Geometry: final body of the model. Coordinates: model frame, mm. A direction names the side the tool comes from. Give positions to 0.01 mm unless a question says otherwise; leave off trailing zeros. Loops run counter-clockwise (first coordinate to the right, second up) from the corner with the lowest first, then second, coordinate; pieces in that order, holes last.
1. Section D-D, the plane z = 5.25. Output: boundary loops of the cut face in (x, y), then the cut area to 3 significant figures.
2. Section B-B, the plane y = 0. Output: boundary loops of the cut face in (x, z).
3. Section A-A, the plane z = 0.5. Output: boundary loops of the cut face in (x, y), then the cut area to 3 significant figures.
4. Section C-C, the plane x = 2.25. Output: boundary loops of the cut face in (y, z), then the cut area to 3 significant figures.
5. Material intervals for line 1 along Z through (x, y) = (2.2, 0); line 2 along Y through (x, z) = (0.9, -0.5); line 3 along Y through (x, z) = (2.8, 6.25), sorted ascending.
6. First-contact query: P1, Ø3, axis at y = 2.5, z = 6, coming from the +X side; P2, Ø1.5, axis at x = 1, z = 6.5, coming from the +Y side; P3, Ø0.5, axis at x = 2, y = 2.5, coming from the +Z side. Flat tips, straight axial feed; report the tip coordinate or a pass-through.
7. Access query for faces 1 (the face through (1.48, -0.04, -2.25)), 2 (the face through (1, 2, 6)), 3 (the face through (1.5, -2.5, 4.574)). Directions: +Z, -Z, +X, -X, +Y, -Y. A direction counts if a zero-diameter tool reaches every point of the face in a straight line with its end or side. Return the directions, or none.
from build123d import *

# Parameters (mm, degrees)
F0_R     = 1.5
F0_W     = 4
F0_H     = 2.9
F1_DEPTH = 3


with BuildPart() as f1:
    # F0 (on Right) → F1 (new body)
    with BuildSketch(Plane.YZ):
        with BuildLine():
            ThreePointArc((2.222473, -0.350876), (2.243108, -0.175977), (2.25, 0))
            ThreePointArc((2.25, 0), (-0.175977, 2.243108), (-2.222473, -0.350876))
            ThreePointArc((-2.222473, -0.350876), (0, -2.25), (2.222473, -0.350876))
        make_face()
        Circle(F0_R, mode=Mode.SUBTRACT)
        with BuildLine():
            ThreePointArc((-2.222473, -0.350876), (-0.175977, 2.243108), (2.25, 0))
            ThreePointArc((2.25, 0), (2.243108, -0.175977), (2.222473, -0.350876))
            Line((2.222473, -0.350876), (3, 4.574038))
            Line((3, 4.574038), (2, 4.574038))
            Line((2, 4.574038), (-2, 4.574038))
            Line((-2, 4.574038), (-3, 4.574038))
            Line((-3, 4.574038), (-2.222473, -0.350876))
        make_face()
        with Locations((0, 6.024038)):
            Rectangle(F0_W, F0_H)
    extrude(amount=F1_DEPTH)


solid = f1.part
Answers below:
1. outline: (0, -2) - (3, -2) - (3, 2) - (0, 2) - close
1. area: 12.0 mm2
2. outline: (0, -2.25) - (3, -2.25) - (3, -1.5) - (0, -1.5) - close; (0, 1.5) - (3, 1.5) - (3, 7.47) - (0, 7.47) - close
3. outline: (0, -2.36) - (3, -2.36) - (3, -1.41) - (0, -1.41) - close; (0, 1.41) - (3, 1.41) - (3, 2.36) - (0, 2.36) - close
3. area: 5.66 mm2
4. outline: (-3, 4.57) - (-2.22, -0.35) arc R2.25 ccw to (2.22, -0.35) - (3, 4.57) - (2, 4.57) - (2, 7.47) - (-2, 7.47) - (-2, 4.57) - close; hole circle Ø3 at (0, 0)
4. area: 36.6 mm2
5. line 1: z = -2.25 to -1.5, 1.5 to 7.47
5. line 2: y = -2.19 to -1.41, 1.41 to 2.19
5. line 3: y = -2 to 2
6. P1: stops at x = 3
6. P2: stops at y = 2
6. P3: stops at z = 4.57
7. face 1: -Z, +X, -X
7. face 2: +Z, +X, -X, +Y
7. face 3: +Z, +X, -X, -Y
